Part model, mm, in its own coordinate system. Face numbers are marked on the shaded views. A direction names the side the tool comes from. Give positions to 0.01 mm unless a question says otherwise; leave off trailing zeros. Loops run counter-clockwise (first coordinate to the right, second up) from the corner with the lowest first, then second, coordinate; pieces in that order, holes last. Notation, with made-up numbers: (-11.5, 50.25) -> (15.5, 50.25) arc R23 ccw to (15.5, 75.25) -> close; hole circle Ø11 at (84, -25). An arc over 180 degrees is marked (long way). One line per question, with ' | ' between items.
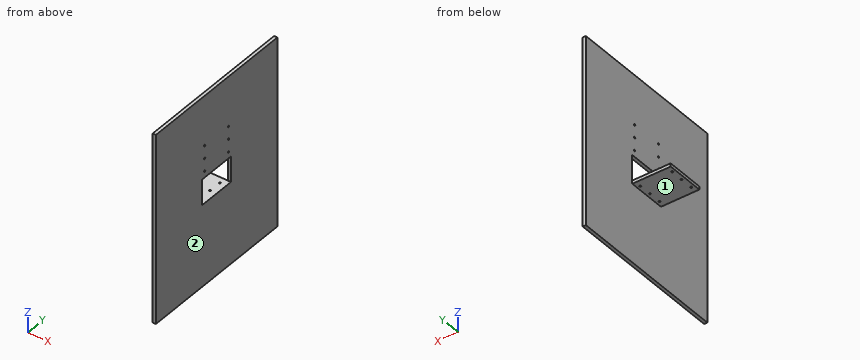
```python
from build123d import *

# Parameters (mm, degrees)
SKETCH_1_W      = 180
SKETCH_1_H      = 180
SKETCH_1_R      = 4
EXTRUDE_1_DEPTH = 15
SKETCH_9_W      = 887.558239328
SKETCH_9_H      = 761.432182166
SKETCH_9_R      = 4
SKETCH_9_W_2    = 120
SKETCH_9_H_2    = 180
EXTRUDE_2_DEPTH = 15


with BuildPart() as part:
    # 草图1 → 凸台-拉伸1 (new body)
    with BuildSketch(Plane.XY):
        Rectangle(SKETCH_1_W, SKETCH_1_H)
        with Locations((-75, 60)):
            Circle(SKETCH_1_R, mode=Mode.SUBTRACT)
        with Locations((-74.035625505, 0)):
            Circle(SKETCH_1_R, mode=Mode.SUBTRACT)
        with Locations((-74.035625505, -60)):
            Circle(SKETCH_1_R, mode=Mode.SUBTRACT)
        with Locations(Location((74.035625505, -60, 0), (0, 0, 180))):
            Circle(SKETCH_1_R, mode=Mode.SUBTRACT)
        with Locations(Location((74.035625505, 0, 0), (0, 0, 180))):
            Circle(SKETCH_1_R, mode=Mode.SUBTRACT)
        with Locations(Location((75, 60, 0), (0, 0, 180))):
            Circle(SKETCH_1_R, mode=Mode.SUBTRACT)
    extrude(amount=EXTRUDE_1_DEPTH)

    # 草图9 → 凸台-拉伸2 (add)
    with BuildSketch(Plane(origin=(90, 0, 0), x_dir=(0, 0, -1), z_dir=(1, 0, 0))):
        with Locations((-75, 0)):
            Rectangle(SKETCH_9_W, SKETCH_9_H)
        with Locations((-165, 75)):
            Circle(SKETCH_9_R, mode=Mode.SUBTRACT)
        with Locations((-225, 75)):
            Circle(SKETCH_9_R, mode=Mode.SUBTRACT)
        with Locations((-285, 75)):
            Circle(SKETCH_9_R, mode=Mode.SUBTRACT)
        with Locations(Location((-285, -75, 0), (0, 0, 180))):
            Circle(SKETCH_9_R, mode=Mode.SUBTRACT)
        with Locations(Location((-225, -75, 0), (0, 0, 180))):
            Circle(SKETCH_9_R, mode=Mode.SUBTRACT)
        with Locations(Location((-165, -75, 0), (0, 0, 180))):
            Circle(SKETCH_9_R, mode=Mode.SUBTRACT)
        with Locations((-75, 0)):
            Rectangle(SKETCH_9_W_2, SKETCH_9_H_2, mode=Mode.SUBTRACT)
    extrude(amount=EXTRUDE_2_DEPTH)


solid = part.part
```
1) Drill centre lines: line 1 (Y direction, x = 99, z = 285); line 2 (Z direction, x = 100, y = -75); line 3 (X direction, y = -142, z = -282). Where is each one in solid material? Low to high.
Found:
line 1: -380.72 to -79, -71 to 71, 79 to 380.72 | line 2: -368.78 to 15, 135 to 161, 169 to 221, 229 to 281, 289 to 518.78 | line 3: 90 to 105
2) Saw through at C-C (z = 251). Give the cut face in (x, y).
Found:
outline: (90, -380.72) -> (105, -380.72) -> (105, 380.72) -> (90, 380.72) -> close
3) Saw through at B-B (x = 36.5). Give the cut face in (y, z), and give its area (3 significant figures).
Found:
outline: (-90, 0) -> (90, 0) -> (90, 15) -> (-90, 15) -> close | area: 2,700 mm2
4) Tool access for the marked faces 1 and 2: list every direction of +Z, -Z, +X, -X, +Y, -Y with a clear straight run to the whole face (end or side of a thin tool).
Found:
face 1: -Z, -X, +Y, -Y | face 2: +Z, -Z, +X, +Y, -Y
5) Pin check, flat tips, straight feed: P1, Ø6.5, axis at x = -74.04, y = -60, coming from the -Z side; P2, Ø8, axis at x = 81, y = -3, coming from the -Z side; P3, Ø10.5, axis at x = -74.04, y = 0, coming from the +Z side; P4, Ø12, axis at x = -39.5, z = 6, coming from the +Y side. Stop position of each tip, or through.
Found:
P1: through | P2: z = 0 | P3: z = 15 | P4: y = 90
6) Saw through at A-A (z = 122.5). Give the cut face in (x, y).
Found:
outline: (90, -380.72) -> (105, -380.72) -> (105, -90) -> (90, -90) -> close; (90, 90) -> (105, 90) -> (105, 380.72) -> (90, 380.72) -> close
